Could you check a few things on this model? Use its own coordinates, in mm. Face numbers are marked on the shaded views. Coordinates: 2 decimals unless noted, no trailing zeros. Order: outer loops, then holes, each group sorted by start corner. A loop starts at its lowest first (then second) coordinate and runs counter-clockwise, first axis right, second up. Notation, with made-up numbers: (-39.75, 89) -> (-35.75, 89) arc R37 cw to (-35.75, 128) -> close; hole circle Ø9 at (-13, 63.25). An arc over 180 degrees is marked (long way). Return JSON: item names as keys, results as strings. Group by question number.
from build123d import *

# Parameters (mm, degrees)
BOSS_EXTRUDE1_DEPTH = 11.5
SKETCH3_R           = 6.171796323
CUT_EXTRUDE1_DEPTH  = 22


with BuildPart() as part:
    # Sketch2 → Boss-Extrude1 (new body, symmetric)
    with BuildSketch(Plane(origin=(0, 0, 0), x_dir=(0, 0, -1), z_dir=(1, 0, 0))):
        with BuildLine():
            Line((-10.5, -13.355315719), (-10.5, 30.769844031))
            Line((-10.5, 30.769844031), (-8.5, 30.769844031))
            Line((-8.5, 30.769844031), (-8.5, -13.355315719))
            ThreePointArc((-8.5, -13.355315719), (0, -21.855315719), (8.5, -13.355315719))
            Line((8.5, -13.355315719), (8.5, 30.769844031))
            Line((8.5, 30.769844031), (10.5, 30.769844031))
            Line((10.5, 30.769844031), (10.5, -13.355315719))
            ThreePointArc((10.5, -13.355315719), (0, -23.855315719), (-10.5, -13.355315719))
        make_face()
    extrude(amount=BOSS_EXTRUDE1_DEPTH, both=True)

    # Sketch3 → Cut-Extrude1 (cut, through all)
    with BuildSketch(Plane.XY.offset(10.5)):
        with Locations((0, 18.082496022)):
            Circle(SKETCH3_R)
    extrude(amount=-CUT_EXTRUDE1_DEPTH, mode=Mode.SUBTRACT)


solid = part.part
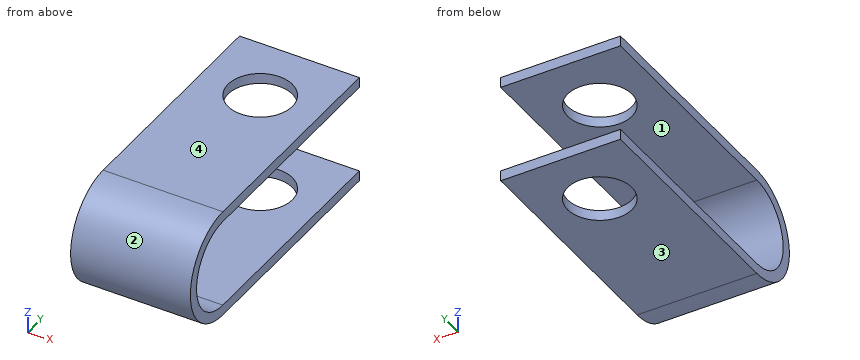
Q1. I want a section at C-C on x = 9. Please give me the cut outline in (y, z).
Q2. We'd pull the mould along Z, two halves only. Please class the marked faces 1, 2, 3 and 4: pulls with the +Z half, pulls with the -Z half, needs draft (parallel to the pull), parting line crosses it, or undercut.
Q3. I need wall thicknesses on line 1 along Z through (x, y) = (-7.25, 17); line 2 along Y through (x, z) = (-0.25, -0.25); line 3 along Y through (x, z) = (0, -9.05). Which ranges of each line are inside material? Lowest first, please. Write a range as from..to.
Q4. I'm going to push flat-ended pins straight in: pin 1 Ø3 at (x, z) = (2.5, 2) entering from +Y; pin 2 Ø7.5 at (x, y) = (0, 18.08) entering from +Z; pin 3 Ø4 at (x, z) = (-7, 3.5) entering from -Y. Where does each tip first touch, or does it pass through?
Q5. I want a section at A-A on y = 5.5. Please give me the cut outline in (x, z).
Q6. I want a section at D-D on y = 21. Please give me the cut outline in (x, z), and give its area (3 significant figures).
Q7. I want a section at B-B on x = 0. Please give me the cut outline in (y, z).
Response values:
{
 "1": {"outline": "(-13.36, -10.5) -> (30.77, -10.5) -> (30.77, -8.5) -> (-13.36, -8.5) arc R8.5 cw to (-13.36, 8.5) -> (30.77, 8.5) -> (30.77, 10.5) -> (-13.36, 10.5) arc R10.5 ccw to start"},
 "2": {"face 1": "undercut", "face 2": "parting line crosses it", "face 3": "pulls with the -Z half", "face 4": "pulls with the +Z half"},
 "3": {"line 1": "z = -10.5..-8.5, 8.5..10.5", "line 2": "y = -23.85..-21.85", "line 3": "y = -18.68..11.91, 24.25..30.77"},
 "4": {"pin 1": "stops at y = -21.1", "pin 2": "passes through", "pin 3": "stops at y = -23.75"},
 "5": {"outline": "(-11.5, -10.5) -> (11.5, -10.5) -> (11.5, -8.5) -> (-11.5, -8.5) -> close; (-11.5, 8.5) -> (11.5, 8.5) -> (11.5, 10.5) -> (-11.5, 10.5) -> close"},
 "6": {"outline": "(-11.5, -10.5) -> (-5.44, -10.5) -> (-5.44, -8.5) -> (-11.5, -8.5) -> close; (-11.5, 8.5) -> (-5.44, 8.5) -> (-5.44, 10.5) -> (-11.5, 10.5) -> close; (5.44, -10.5) -> (11.5, -10.5) -> (11.5, -8.5) -> (5.44, -8.5) -> close; (5.44, 8.5) -> (11.5, 8.5) -> (11.5, 10.5) -> (5.44, 10.5) -> close", "area": "48.5 mm²"},
 "7": {"outline": "(-13.36, -10.5) -> (11.91, -10.5) -> (11.91, -8.5) -> (-13.36, -8.5) arc R8.5 cw to (-13.36, 8.5) -> (11.91, 8.5) -> (11.91, 10.5) -> (-13.36, 10.5) arc R10.5 ccw to start; (24.25, -10.5) -> (30.77, -10.5) -> (30.77, -8.5) -> (24.25, -8.5) -> close; (24.25, 8.5) -> (30.77, 8.5) -> (30.77, 10.5) -> (24.25, 10.5) -> close"}
}
